Autodesk Inventor part; units mm, degrees
ref_plane "YZ Plane" through (0, 0, 0) normal (1, 0, 0) x (0, 1, 0)
ref_plane "XZ Plane" through (0, 0, 0) normal (0, 1, 0) x (-1, 0, 0)
ref_plane "XY Plane" through (0, 0, 0) normal (0, 0, 1) x (1, 0, 0)
sketch "Sketch1" plane through (0, 0, 0) normal (0, 0, 1) x (1, 0, 0)
  circle A0 centre (0, 0) radius 13.825
  circle A1 centre (0, 0) radius 12.625
  dimension "d0" = 27.65
  dimension "d1" = 25.25
extrude "Extrusion1" add sketch "Sketch1" along normal blind 1.8
sketch "Sketch2" plane through (0, 0, 1.8) normal (0, 0, 1) x (1, 0, 0)
  circle A0 centre (0, 0) radius 12.625
  circle A1 centre (0, 0) radius 14.775
  dimension "d5" = 29.55
  dimension "d16" = 25.25
extrude "Extrusion2" add sketch "Sketch2" along normal blind 1.2
sketch "Sketch3" plane through (0, 0, 0) normal (0, 0, 1) x (1, 0, 0)
  line L0 (11.2898, 0.9) -> (17.9351, 0.9)
  line L1 (17.9351, 0.9) -> (17.9351, -0.9)
  line L2 (17.9351, -0.9) -> (11.2898, -0.9)
  line L3 (11.2898, -0.9) -> (11.2898, 0.9)
  point P0 (0, 0)
  dimension "d13" = 1.8
  dimension "d14" = 6.6453
  dimension "d15" = 0.9
extrude "Extrusion3" cut sketch "Sketch3" along normal blind 6
chamfer "Chamfer1" distance 0.5 angle 45 1 edges at (-13.825, 0, 1.8)
mirror "Mirror2" about plane through (0, 0, 0) normal (0, 0, 1) of "Extrusion1", "Extrusion2", "Extrusion3", "Chamfer1"
fillet "Fillet1" radius 0.5 11 edges at (-12.625, 0, 3) (-12.625, 0, -3) (12.5929, -0.9, 0) (13.6702, -0.9, 3) (13.6702, -0.9, -3) (13.6702, 0.9, 3) (13.6702, 0.9, -3) (14.7476, 0.9, 2.4) (14.7476, 0.9, -2.4) (14.7476, -0.9, -2.4) (14.7476, -0.9, 2.4)
equation "\"d16\" = d1"
properties part number "maxtubingBoreWireProtectInsert"
The model under review builds one solid part; all positions refer to its coordinate system, in mm. A direction names the side the tool comes from. Round coordinates to 2 decimals unless told otherwise and drop trailing zeros. Order: outer loops, then holes, each group sorted by start corner. A loop starts at its lowest first (then second) coordinate and runs counter-clockwise, first axis right, second up.
Item 1: For pin 1 (2 mm diameter, centred on x = 10.5, z = -1, fed in from +Y); pin 2 (2 mm diameter, centred on y = 11, z = -1.5, fed in from -X), all flat-tipped, find the tip position at first contact; note any pin that passes through.
Working result:
pin 1: stops at y = 10.97
pin 2: stops at x = -10.83
Item 2: Add section B-B, the plane y = 0. State the section outline as (x, z) points (3 decimals), and give its area (3 significant figures).
Working result:
outline: (-14.775, -3) - (-13.125, -3) arc R0.5 ccw to (-12.625, -2.5) - (-12.625, 2.5) arc R0.5 ccw to (-13.125, 3) - (-14.775, 3) - (-14.775, 1.8) - (-14.325, 1.8) - (-13.825, 1.3) - (-13.825, -1.3) - (-14.325, -1.8) - (-14.775, -1.8) - close
area: 9.62 mm2
Item 3: Draft analysis for pull direction Z (two halves, no side actions). For faces 4 (the conical face through (-13.95, 0.6, 1.44)), 5 (the cylindrical face through (-13.81, 0.6, 0.02)), 6 (the flat face through (-9, -10, 3)), 7 (the cylindrical face through (-14.76, -0.63, 2.39)), state which applies: released by +Z, released by -Z, zero draft, split by the parting line, or undercut.
Working result:
face 4: undercut
face 5: undercut
face 6: released by +Z
face 7: zero draft
Item 4: To check wall thickness, follow probe 1 along Y at (x, z) = (0, 0.6) (3 decimals); probe 2 along Y at (x, z) = (-7.75, -1.5); probe 3 along X at (y, z) = (-10.5, -0.25). State the ranges of each line that lie inside material, in increasing order.
Working result:
probe 1: y = -13.825 to -12.625, 12.625 to 13.825
probe 2: y = -11.69 to -9.97, 9.97 to 11.69
probe 3: x = -8.99 to -7.01, 7.01 to 8.99
Item 5: Add section A-A, the plane x = 0. State the section outline as (y, z) points (3 decimals).
Working result:
outline: (-14.775, -3) - (-13.125, -3) arc R0.5 ccw to (-12.625, -2.5) - (-12.625, 2.5) arc R0.5 ccw to (-13.125, 3) - (-14.775, 3) - (-14.775, 1.8) - (-14.325, 1.8) - (-13.825, 1.3) - (-13.825, -1.3) - (-14.325, -1.8) - (-14.775, -1.8) - close; (12.625, -2.5) arc R0.5 ccw to (13.125, -3) - (14.775, -3) - (14.775, -1.8) - (14.325, -1.8) - (13.825, -1.3) - (13.825, 1.3) - (14.325, 1.8) - (14.775, 1.8) - (14.775, 3) - (13.125, 3) arc R0.5 ccw to (12.625, 2.5) - close
Item 6: Machinability: for faces 1 (the flat face through (13, 0.9, 0)), 2 (the flat face through (-10, 9, -3)), 3 (the conical face through (-13.95, -0.6, -1.44)), which of the approach directions +Z, -Z, +X, -X, +Y, -Y give a long, thin tool a straight path to every point of the face, cutting with its end or side? Answer none if there is none.
Working result:
face 1: +Z, -Z, +X
face 2: -Z, +X, -X, +Y, -Y
face 3: none
Item 7: Add section C-C, the plane z = -0.5. State the section outline as (x, y) points (3 decimals), and give its area (3 significant figures).
Working result:
outline: (12.553, -1.347) arc R12.625 cw (long way) to (12.593, 0.9) - (13.796, 0.9) arc R13.825 ccw (long way) to (13.796, -0.9) - (13.05, -0.9) arc R0.5 ccw to start
area: 97.5 mm2
